from build123d import *

# Parameters (mm, degrees)
ESBO_O1_W                = 3
ESBO_O1_H                = 10
ESBO_O1_W_2              = 6
RESSALTO_EXTRUS_O1_DEPTH = 3


with BuildPart() as part:
    # Esboço1 → Ressalto-extrusão1 (new body)
    with BuildSketch(Plane.XY):
        Polygon((-12, -5), (-12, -7.5), (12, -7.5), (12, -5), (12, 5), (12, 7.5), (-12, 7.5), (-12, 5), align=None)
        with Locations((-13.5, 0)):
            Rectangle(ESBO_O1_W, ESBO_O1_H)
        with Locations((15, 0)):
            Rectangle(ESBO_O1_W_2, ESBO_O1_H)
        Polygon((18, 5), (18, -5), (18, -10), (26, -10), (26, 10), (18, 10), align=None)
    extrude(amount=RESSALTO_EXTRUS_O1_DEPTH)


solid = part.part
Geometry check sheet. Reference: the model listing, model coordinates, mm. A direction names the side the tool comes from. Round coordinates to 2 decimals unless told otherwise and drop trailing zeros. Loops run counter-clockwise (first coordinate to the right, second up) from the corner with the lowest first, then second, coordinate; pieces in that order, holes last. Notation, with made-up numbers: (-26.75, 65) - (-16.75, 65) arc R14 cw to (-16.75, 75) - close; hole circle Ø5 at (25, 6.5). An arc over 180 degrees is marked (long way). Answer as CSV lines item,"result".
(1) Cross-section at A-A, the plane y = -6.25. Enter the section's corners in (x, z).
Output values:
outline,"(-12, 0) - (12, 0) - (12, 3) - (-12, 3) - close; (18, 0) - (26, 0) - (26, 3) - (18, 3) - close"
(2) Depth check by flat-ended pin: pin 1 Ø4 at (x, y) = (2.5, 0) entering from -Z; pin 2 Ø1.5 at (x, z) = (14, 2) entering from -Y; pin 3 Ø0.9 at (x, z) = (14.5, 1.5) entering from +Y; pin 4 Ø0.9 at (y, z) = (7, 2) entering from -X. Enter the tip coordinate at first touch or a pass-through.
Output values:
pin 1,"stops at z = 0"
pin 2,"stops at y = -5"
pin 3,"stops at y = 5"
pin 4,"stops at x = -12"
(3) Cross-section at B-B, the plane z = 1.75. Enter the section's corners in (x, y), and give its area (3 significant figures).
Output values:
outline,"(-15, -5) - (-12, -5) - (-12, -7.5) - (12, -7.5) - (12, -5) - (18, -5) - (18, -10) - (26, -10) - (26, 10) - (18, 10) - (18, 5) - (12, 5) - (12, 7.5) - (-12, 7.5) - (-12, 5) - (-15, 5) - close"
area,"610 mm²"
(4) Set-up check for faces 5 (the face through (15, -5, 1)), 6 (the face through (0, -7.5, 1)), 7 (the face through (0, 7.5, 1)), 8 (the face through (12, 6, 1)): record each of +Z, -Z, +X, -X, +Y, -Y from which the full face is reachable in a straight line by a thin tool's end or side.
Output values:
face 5,"+Z, -Z, -Y"
face 6,"+Z, -Z, -X, -Y"
face 7,"+Z, -Z, -X, +Y"
face 8,"+Z, -Z, +Y"
(5) Cross-section at C-C, the plane y = -9. Enter the section's corners in (x, z), and give its area (3 significant figures).
Output values:
outline,"(18, 0) - (26, 0) - (26, 3) - (18, 3) - close"
area,"24.0 mm²"
(6) Material ranges on line 1 along X through (y, z) = (-6.75, 2.6); line 2 along Y through (x, z) = (17.5, 0.25); line 3 along Y through (x, z) = (-1.5, 2.15), recorded low to high.
Output values:
line 1,"x = -12 to 12, 18 to 26"
line 2,"y = -5 to 5"
line 3,"y = -7.5 to 7.5"
(7) Cross-section at D-D, the plane x = 7.5. Enter the section's corners in (y, z), and give its area (3 significant figures).
Output values:
outline,"(-7.5, 0) - (7.5, 0) - (7.5, 3) - (-7.5, 3) - close"
area,"45.0 mm²"
(8) Release check for a two-part mould opening along X. For faces 1 (the face through (12, -6, 1)), 2 (the face through (22, -10, 1)), 3 (the face through (15, 5, 1)), 4 (the face through (-12, 6, 1)) record: released by +X, released by -X, zero draft, split by the parting line, or undercut.
Output values:
face 1,"undercut"
face 2,"zero draft"
face 3,"undercut"
face 4,"released by -X"
